Design review of the part built by this model. Coordinates are the model's own, in mm. A direction names the side the tool comes from. Give positions to 0.01 mm unless a question says otherwise; leave off trailing zeros. Order: outer loops, then holes, each group sorted by start corner. A loop starts at its lowest first (then second) coordinate and runs counter-clockwise, first axis right, second up. Notation, with made-up numbers: (-34.75, 73) -> (-25.75, 73) arc R14 cw to (-25.75, 84) -> close; hole circle Ø7 at (56, 29.5). An arc over 180 degrees is marked (long way). One line per item, written item: value.
Autodesk Inventor part; units mm, degrees
ref_plane "YZ Plane" through (0, 0, 0) normal (1, 0, 0) x (0, 1, 0)
ref_plane "XZ Plane" through (0, 0, 0) normal (0, 1, 0) x (-1, 0, 0)
ref_plane "XY Plane" through (0, 0, 0) normal (0, 0, 1) x (1, 0, 0)
sketch "Sketch1" plane through (0, 0, 0) normal (0, 0, 1) x (1, 0, 0)
  line L0 (0, 0) -> (0, 460.0937) construction
  line L1 (-342.9, 0) -> (-420.0646, 0)
  line L2 (-420.0646, 0) -> (-420.0646, 1.5875)
  line L3 (-420.0646, 1.5875) -> (-342.9, 1.5875)
  line L4 (-342.9, 1.5875) -> (-342.9, 0)
  line L5 (-342.9, 1.5875) -> (-517.525, 1.5875)
  line L6 (-517.525, 1.5875) -> (-517.525, 96.8375)
  line L7 (-517.525, 96.8375) -> (-342.9, 96.8375)
  line L8 (-342.9, 96.8375) -> (-342.9, 1.5875)
  line L9 (-342.9, 96.8375) -> (-342.9, 206.248)
  line L10 (-342.9, 206.248) -> (-355.6, 206.248)
  line L11 (-355.6, 206.248) -> (-391.287, 96.8375)
  dimension "d0" = 342.9
  dimension "d2" = 95.25
  dimension "d3" = 1.5875
  dimension "d4" = 517.525
  dimension "d5" = 206.248
  dimension "d6" = 391.287
  dimension "d7" = 355.6
revolve "Revolution1" add sketch "Sketch1" angle 360 about axis through (0, 0, 0) along (0, 1, 0)
properties part number "A1-19037-100-XX 28in CL300 Slip on Flange"
Item 1: To check wall thickness, follow line 1 along Z through (x, y) = (136, 100.5); line 2 along Z through (x, y) = (-122, 39.5); line 3 along X through (y, z) = (44, -149). State the ranges of each line that lie inside material, in increasing order. Write a range as from..to.
Returned:
line 1: -365.62..-314.78, 314.78..365.62
line 2: -502.94..-320.46, 320.46..502.94
line 3: -495.61..-308.84, 308.84..495.61
Item 2: Add section B-B on z = 0. Give the boundary of the cut face in (x, y) (1 decimal).
Returned:
outline: (-517.5, 1.6) -> (-420.1, 1.6) -> (-420.1, 0) -> (-342.9, 0) -> (-342.9, 206.2) -> (-355.6, 206.2) -> (-391.3, 96.8) -> (-517.5, 96.8) -> close; (342.9, 0) -> (420.1, 0) -> (420.1, 1.6) -> (517.5, 1.6) -> (517.5, 96.8) -> (391.3, 96.8) -> (355.6, 206.2) -> (342.9, 206.2) -> close
Item 3: Machinability: for faces 1 (the cylindrical face through (-400.667, 0.805, 126.176)), 2 (the conical face through (-341.31, 199.4, -107.48)), which of the approach directions +Z, -Z, +X, -X, +Y, -Y give a long, thin tool a straight path to every point of the face, cutting with its end or side? Answer none if there is none.
Returned:
face 1: -Y
face 2: +Y
Item 4: Draft analysis for pull direction X (two halves, no side actions). For faces 3 (the cylindrical face through (112.19, 49.88, -505.22)), 4 (the cylindrical face through (-184.341, 101.68, -289.135)), 5 (the flat face through (-74, 96.838, 386)), state which applies: pulls with the +X half, pulls with the -X half, needs draft (parallel to the pull), parting line crosses it, or undercut.
Returned:
face 3: parting line crosses it
face 4: undercut
face 5: needs draft
Item 5: Add section A-A on x = 0. Give the boundary of the cut face in (y, z) (1 decimal), plus the area to 3 significant figures.
Returned:
outline: (0, -420.1) -> (1.6, -420.1) -> (1.6, -517.5) -> (96.8, -517.5) -> (96.8, -391.3) -> (206.2, -355.6) -> (206.2, -342.9) -> (0, -342.9) -> close; (0, 342.9) -> (206.2, 342.9) -> (206.2, 355.6) -> (96.8, 391.3) -> (96.8, 517.5) -> (1.6, 517.5) -> (1.6, 420.1) -> (0, 420.1) -> close
area: 40,200 mm²
Item 6: Add section D-D on y = 37.5. Give the boundary of the cut face in (x, z) (3 decimals), plus the area to 3 significant figures.
Returned:
outline: circle Ø1035.05 at (0, 0); hole circle Ø685.8 at (0, 0)
area: 472,000 mm²
Item 7: Clearance check with flat-ended pins moving along their axes: P1, Ø4, axis at y = 117.5, z = 202, coming from the -X side; P2, Ø12, axis at x = 188, y = 34, coming from the -Z side; P3, Ø5, axis at x = -142.5, y = 181.5, coming from the +Z side. State where each tip first meets the part, or that it passes through.
Returned:
P1: x = -328.67
P2: z = -484.47
P3: z = 335.97
